The drawing under review shows one solid part. Ordinate dimensions are in mm from its lowest x, y, z. Coordinates: 2 decimals unless noted, no trailing zeros. Loops run counter-clockwise (first coordinate to the right, second up) from the corner with the lowest first, then second, coordinate; pieces in that order, holes last. Notation, with made-up numbers: M 57,-8 L 99,-8 A21 ccw 99,22 Z; hole C 33.5,-12.75 d7. An arc over 180 degrees is marked long. Put each result on its own line as item: value.
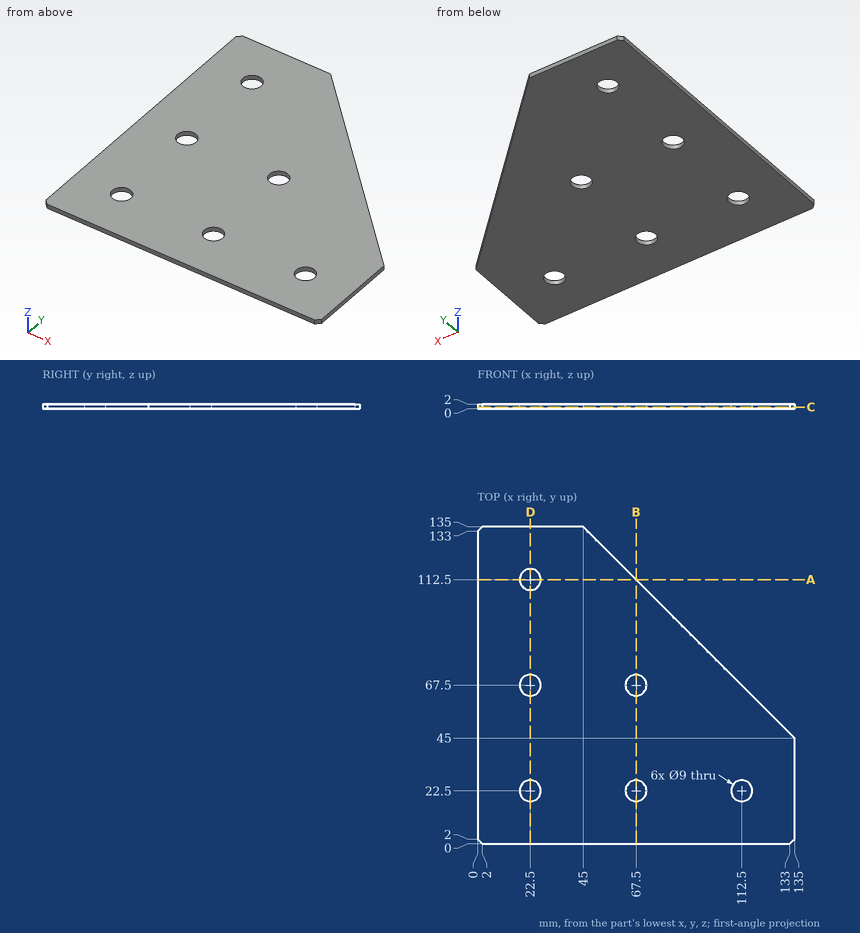
(1) Add section C-C (z = 0.7). Write out the cut boundary in (x, y).
Determined:
outline: M 0,2 L 2,0 L 133,0 L 135,2 L 135,45 L 45,135 L 2,135 L 0,133 Z; hole C 22.5,22.5 d9; hole C 22.5,67.5 d9; hole C 22.5,112.5 d9; hole C 67.5,22.5 d9; hole C 67.5,67.5 d9; hole C 112.5,22.5 d9
(2) Add section B-B (x = 67.5). Write out the cut boundary in (y, z), plus the area to 3 significant figures.
Determined:
outline: M 0,0 L 18,0 L 18,2 L 0,2 Z; M 27,0 L 63,0 L 63,2 L 27,2 Z; M 72,0 L 112.5,0 L 112.5,2 L 72,2 Z
area: 189 mm^2
(3) For pin 1 (11.5 mm diameter, centred on x = 22.5, y = 67.5, fed in from +Z), flat-tipped, find the tip position at first contact; note if it passes through.
Determined:
pin 1: stops at z = 2
(4) Add section A-A (y = 112.5). Write out the cut boundary in (x, z), plus the area to 3 significant figures.
Determined:
outline: M 0,0 L 18,0 L 18,2 L 0,2 Z; M 27,0 L 67.5,0 L 67.5,2 L 27,2 Z
area: 117 mm^2
(5) Add section D-D (x = 22.5). Write out the cut boundary in (y, z), plus the area to 3 significant figures.
Determined:
outline: M 0,0 L 18,0 L 18,2 L 0,2 Z; M 27,0 L 63,0 L 63,2 L 27,2 Z; M 72,0 L 108,0 L 108,2 L 72,2 Z; M 117,0 L 135,0 L 135,2 L 117,2 Z
area: 216 mm^2
(6) Wall thickness on line 1 along X through (y, z) = (22.5, 1.65); line 2 along Y through (x, z) = (67.5, 0.5): over which ranges is each line inside the solid? List them lowest first. Write a range as [from, to].
Determined:
line 1: x = [0, 18], [27, 63], [72, 108], [117, 135]
line 2: y = [0, 18], [27, 63], [72, 112.5]
